from build123d import *

# Parameters (mm, degrees)
CROQUIS1_R              = 3.35
SALIENTE_EXTRUIR1_DEPTH = 146.6


with BuildPart() as part:
    # Croquis1 → Saliente-Extruir1 (new body)
    with BuildSketch(Plane.XY):
        with BuildLine():
            Line((-12.05, -30.05), (-4, -30.05))
            Line((-4, -30.05), (-4, -27.75))
            Line((-4, -27.75), (-11.7, -27.75))
            Line((-11.7, -27.75), (-5, -21.05))
            Line((-5, -21.05), (5, -21.05))
            Line((5, -21.05), (11.7, -27.75))
            Line((11.7, -27.75), (4, -27.75))
            Line((4, -27.75), (4, -30.05))
            Line((4, -30.05), (12.05, -30.05))
            ThreePointArc((12.05, -30.05), (14.171320344, -29.171320344), (15.05, -27.05))
            Line((15.05, -27.05), (15.05, -18.55))
            Line((15.05, -18.55), (12.75, -18.55))
            Line((12.75, -18.55), (12.75, -25.8))
            Line((12.75, -25.8), (6.5, -19.55))
            Line((6.5, -19.55), (6.5, -9.55))
            Line((6.5, -9.55), (12.75, -3.3))
            Line((12.75, -3.3), (12.75, -10.55))
            Line((12.75, -10.55), (15.05, -10.55))
            Line((15.05, -10.55), (15.05, 10.55))
            Line((15.05, 10.55), (12.75, 10.55))
            Line((12.75, 10.55), (12.75, 3.3))
            Line((12.75, 3.3), (6.5, 9.55))
            Line((6.5, 9.55), (6.5, 19.55))
            Line((6.5, 19.55), (12.75, 25.8))
            Line((12.75, 25.8), (12.75, 18.55))
            Line((12.75, 18.55), (15.05, 18.55))
            Line((15.05, 18.55), (15.05, 27.05))
            ThreePointArc((15.05, 27.05), (14.171320344, 29.171320344), (12.05, 30.05))
            Line((12.05, 30.05), (4, 30.05))
            Line((4, 30.05), (4, 27.75))
            Line((4, 27.75), (11.7, 27.75))
            Line((11.7, 27.75), (5, 21.05))
            Line((5, 21.05), (-5, 21.05))
            Line((-5, 21.05), (-11.7, 27.75))
            Line((-11.7, 27.75), (-4, 27.75))
            Line((-4, 27.75), (-4, 30.05))
            Line((-4, 30.05), (-12.05, 30.05))
            ThreePointArc((-12.05, 30.05), (-14.171320344, 29.171320344), (-15.05, 27.05))
            Line((-15.05, 27.05), (-15.05, 18.55))
            Line((-15.05, 18.55), (-12.75, 18.55))
            Line((-12.75, 18.55), (-12.75, 25.8))
            Line((-12.75, 25.8), (-6.5, 19.55))
            Line((-6.5, 19.55), (-6.5, 9.55))
            Line((-6.5, 9.55), (-12.75, 3.3))
            Line((-12.75, 3.3), (-12.75, 10.55))
            Line((-12.75, 10.55), (-15.05, 10.55))
            Line((-15.05, 10.55), (-15.05, -10.55))
            Line((-15.05, -10.55), (-12.75, -10.55))
            Line((-12.75, -10.55), (-12.75, -3.3))
            Line((-12.75, -3.3), (-6.5, -9.55))
            Line((-6.5, -9.55), (-6.5, -19.55))
            Line((-6.5, -19.55), (-12.75, -25.8))
            Line((-12.75, -25.8), (-12.75, -18.55))
            Line((-12.75, -18.55), (-15.05, -18.55))
            Line((-15.05, -18.55), (-15.05, -27.05))
            ThreePointArc((-15.05, -27.05), (-14.171320344, -29.171320344), (-12.05, -30.05))
        make_face()
        with Locations((0, 14.55)):
            Circle(CROQUIS1_R, mode=Mode.SUBTRACT)
        with Locations((0, -14.55)):
            Circle(CROQUIS1_R, mode=Mode.SUBTRACT)
        Polygon((-5, 8.05), (5, 8.05), (11.7, 1.35), (12.75, 0.3), (12.75, -0.3), (11.7, -1.35), (5, -8.05), (-5, -8.05), (-11.7, -1.35), (-12.75, -0.3), (-12.75, 0.3), (-11.7, 1.35), align=None, mode=Mode.SUBTRACT)
    extrude(amount=SALIENTE_EXTRUIR1_DEPTH)


solid = part.part
CAD build for the part. Positions are in the model's coordinates, mm. A direction names the side the tool comes from. Give positions to 0.01 mm unless a question says otherwise; leave off trailing zeros. Order: outer loops, then holes, each group sorted by start corner. A loop starts at its lowest first (then second) coordinate and runs counter-clockwise, first axis right, second up. Notation, with made-up numbers: (-38.75, 89) - (10.25, 89) arc R24 ccw to (10.25, 99) - close; hole circle Ø1 at (64, -24). An arc over 180 degrees is marked (long way). Answer in a Markdown table with one row per item.
1. Probe probe 1 along Y at (x, z) = (0, 115); probe 2 along Y at (x, z) = (-5.5, 107); probe 3 along X at (y, z) = (-15, 39.5). List the from-to ranges inside material, lowest first. Write a range as [from, to].
Data:
| item | result |
|---|---|
| probe 1 | y = [-21.05, -17.9], [-11.2, -8.05], [8.05, 11.2], [17.9, 21.05] |
| probe 2 | y = [-30.05, -27.75], [-21.55, -7.55], [7.55, 21.55], [27.75, 30.05] |
| probe 3 | x = [-6.5, -3.32], [3.32, 6.5] |
2. Saw through at C-C, the plane x = 9. Give the cut face in (y, z), plus the area to 3 significant figures.
Data:
| item | result |
|---|---|
| outline | (-30.05, 0) - (-27.75, 0) - (-27.75, 146.6) - (-30.05, 146.6) - close; (-25.05, 0) - (-22.05, 0) - (-22.05, 146.6) - (-25.05, 146.6) - close; (-7.05, 0) - (-4.05, 0) - (-4.05, 146.6) - (-7.05, 146.6) - close; (4.05, 0) - (7.05, 0) - (7.05, 146.6) - (4.05, 146.6) - close; (22.05, 0) - (25.05, 0) - (25.05, 146.6) - (22.05, 146.6) - close; (27.75, 0) - (30.05, 0) - (30.05, 146.6) - (27.75, 146.6) - close |
| area | 2,430 mm² |
3. Tool access for faces 1 (the flat face through (15.05, 23, 72)), 2 (the flat face through (0, -8.05, 72)): list every direction of +Z, -Z, +X, -X, +Y, -Y with a clear straight run to the whole face (end or side of a thin tool).
Data:
| item | result |
|---|---|
| face 1 | +Z, -Z, +X, +Y, -Y |
| face 2 | +Z, -Z |
4. Saw through at A-A, the plane x = 0. Give the cut face in (y, z), plus the area to 3 significant figures.
Data:
| item | result |
|---|---|
| outline | (-21.05, 0) - (-17.9, 0) - (-17.9, 146.6) - (-21.05, 146.6) - close; (-11.2, 0) - (-8.05, 0) - (-8.05, 146.6) - (-11.2, 146.6) - close; (8.05, 0) - (11.2, 0) - (11.2, 146.6) - (8.05, 146.6) - close; (17.9, 0) - (21.05, 0) - (21.05, 146.6) - (17.9, 146.6) - close |
| area | 1,850 mm² |
5. Saw through at B-B, the plane y = 14.55. Give the cut face in (x, z), plus the area to 3 significant figures.
Data:
| item | result |
|---|---|
| outline | (-6.5, 0) - (-3.35, 0) - (-3.35, 146.6) - (-6.5, 146.6) - close; (3.35, 0) - (6.5, 0) - (6.5, 146.6) - (3.35, 146.6) - close |
| area | 924 mm² |
6. Pull direction Y, two halves, no side cores. Call faces 3 (the flat face through (-8.4, -24.45, 72.27)), 4 (the flat face through (-15.05, 0, 72)), 5 (the cylindrical face through (14.15, -29.19, 72.27)): pulls with the +Y half, pulls with the -Y half, needs draft (parallel to the pull), parting line crosses it, or undercut.
Data:
| item | result |
|---|---|
| face 3 | undercut |
| face 4 | needs draft |
| face 5 | pulls with the -Y half |
7. Flat gauge pins, fed straight in: pin 1 (2.5 mm diameter, centred on y = -28.5, z = 63.5, fed in from +X); pin 2 (1.2 mm diameter, centred on x = 13.5, z = 52.5, fed in from -Y); pin 3 (1.8 mm diameter, centred on x = 13.5, z = 86, fed in from +Y). Where does each tip first touch, or does it go through?
Data:
| item | result |
|---|---|
| pin 1 | stops at x = 15.04 |
| pin 2 | stops at y = -29.93 |
| pin 3 | stops at y = 30 |
8. Saw through at D-D, the plane z = 107. Count the separate pieces of the cut face and the enclosed holes in it, plus the area to 3 significant figures.
Data:
| item | result |
|---|---|
| separate pieces | 1 |
| enclosed holes | 3 |
| area | 700 mm² |
